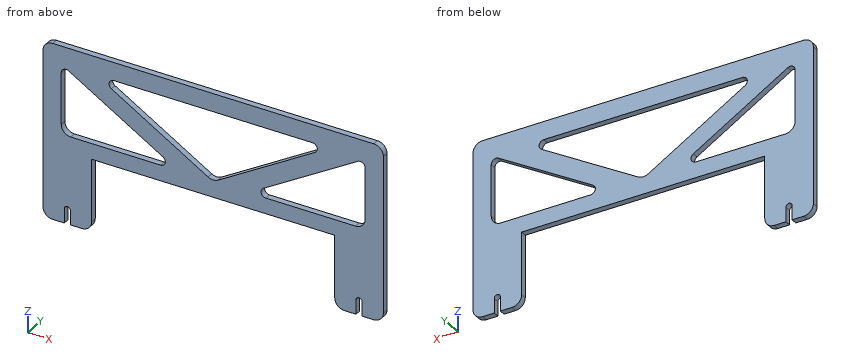
from build123d import *

# Parameters (mm, degrees)
SKETCH1_W           = 177.8
SKETCH1_H           = 67.31
BOSS_EXTRUDE1_DEPTH = 3.175
CUT_EXTRUDE1_DEPTH  = 4.175
CUT_EXTRUDE2_DEPTH  = 4.175
SKETCH5_W           = 127
SKETCH5_H           = 12.7
CUT_EXTRUDE3_DEPTH  = 4.175
FILLET1_R           = 5.08
FILLET2_R           = 2.54
SKETCH7_W           = 25.4
SKETCH7_H           = 38.1
BOSS_EXTRUDE2_DEPTH = 3.175
CUT_EXTRUDE4_DEPTH  = 4.175
FILLET3_R           = 5.08


with BuildPart() as part:
    # Sketch1 → Boss-Extrude1 (new body)
    with BuildSketch(Plane(origin=(0, 0, 0), x_dir=(1, 0, 0), z_dir=(0, 1, 0))):
        with Locations((88.9, 33.655)):
            Rectangle(SKETCH1_W, SKETCH1_H)
    extrude(amount=BOSS_EXTRUDE1_DEPTH)

    # Sketch3 → Cut-Extrude1 (cut, through all)
    with BuildSketch(Plane(origin=(0, 3.175, 0), x_dir=(1, 0, 0), z_dir=(0, 1, 0))):
        Polygon((88.9, 46.355), (27.943666175, 9.525), (149.856333825, 9.525), align=None)
        Polygon((9.525, 46.355), (9.525, 9.525), (70.481333825, 46.355), align=None)
        Polygon((168.275, 9.525), (107.318666175, 46.355), (168.275, 46.355), align=None)
    extrude(amount=-CUT_EXTRUDE1_DEPTH, mode=Mode.SUBTRACT)

    # Sketch4 → Cut-Extrude2 (cut, through all)
    with BuildSketch(Plane(origin=(0, 3.175, 0), x_dir=(1, 0, 0), z_dir=(0, 1, 0))):
        with BuildLine():
            Line((11.1125, 67.31), (11.1125, 62.23))
            ThreePointArc((11.1125, 62.23), (12.7, 60.6425), (14.2875, 62.23))
            Line((14.2875, 62.23), (14.2875, 67.31))
            Line((14.2875, 67.31), (11.1125, 67.31))
        make_face()
        with BuildLine():
            Line((166.6875, 67.31), (166.6875, 62.23))
            ThreePointArc((166.6875, 62.23), (165.1, 60.6425), (163.5125, 62.23))
            Line((163.5125, 62.23), (163.5125, 67.31))
            Line((163.5125, 67.31), (166.6875, 67.31))
        make_face()
    extrude(amount=-CUT_EXTRUDE2_DEPTH, mode=Mode.SUBTRACT)

    # Sketch5 → Cut-Extrude3 (cut, through all)
    with BuildSketch(Plane(origin=(0, 3.175, 0), x_dir=(1, 0, 0), z_dir=(0, 1, 0))):
        with Locations((88.9, 60.96)):
            Rectangle(SKETCH5_W, SKETCH5_H)
    extrude(amount=-CUT_EXTRUDE3_DEPTH, mode=Mode.SUBTRACT)

    # Fillet1
    fillet1_edges = [part.edges().sort_by_distance(p)[0] for p in [
        (88.9, 1.5875, -46.355),
        (9.525, 1.5875, -46.355),
        (168.275, 1.5875, -46.355),
        (0, 1.5875, -67.31),
        (177.8, 1.5875, -67.31),
        (177.8, 1.5875, 0),
        (0, 1.5875, 0),
        (25.4, 1.5875, -67.31),
        (152.4, 1.5875, -67.31),
    ]]
    fillet(fillet1_edges, radius=FILLET1_R)

    # Fillet2
    fillet2_edges = [part.edges().sort_by_distance(p)[0] for p in [
        (149.856333825, 1.5875, -9.525),
        (27.943666175, 1.5875, -9.525),
        (70.481333825, 1.5875, -46.355),
        (9.525, 1.5875, -9.525),
        (168.275, 1.5875, -9.525),
        (107.318666175, 1.5875, -46.355),
    ]]
    fillet(fillet2_edges, radius=FILLET2_R)

    # Sketch7 → Boss-Extrude2 (add)
    with BuildSketch(Plane(origin=(0, 3.175, 0), x_dir=(1, 0, 0), z_dir=(0, 1, 0))):
        with Locations((12.7, 73.66)):
            Rectangle(SKETCH7_W, SKETCH7_H)
        with Locations((165.1, 73.66)):
            Rectangle(SKETCH7_W, SKETCH7_H)
    extrude(amount=-BOSS_EXTRUDE2_DEPTH)

    # Sketch8 → Cut-Extrude4 (cut, through all)
    with BuildSketch(Plane(origin=(0, 3.175, 0), x_dir=(1, 0, 0), z_dir=(0, 1, 0))):
        with BuildLine():
            Line((11.1125, 92.71), (11.1125, 85.09))
            ThreePointArc((11.1125, 85.09), (12.7, 83.5025), (14.2875, 85.09))
            Line((14.2875, 85.09), (14.2875, 92.71))
            Line((14.2875, 92.71), (11.1125, 92.71))
        make_face()
        with BuildLine():
            Line((163.5125, 85.09), (163.5125, 92.71))
            Line((163.5125, 92.71), (166.6875, 92.71))
            Line((166.6875, 92.71), (166.6875, 85.09))
            ThreePointArc((166.6875, 85.09), (165.1, 83.5025), (163.5125, 85.09))
        make_face()
    extrude(amount=-CUT_EXTRUDE4_DEPTH, mode=Mode.SUBTRACT)

    # Fillet3
    fillet3_edges = [part.edges().sort_by_distance(p)[0] for p in [
        (25.4, 1.5875, -92.71),
        (0, 1.5875, -92.71),
        (177.8, 1.5875, -92.71),
        (152.4, 1.5875, -92.71),
    ]]
    fillet(fillet3_edges, radius=FILLET3_R)


solid = part.part
Build history of the part. All positions in model axes, mm. Round coordinates to 2 decimals unless told otherwise and drop trailing zeros. Loops run counter-clockwise (first coordinate to the right, second up) from the corner with the lowest first, then second, coordinate; pieces in that order, holes last. Notation, with made-up numbers: (-31.5, 70) -> (25.5, 70) arc R13 cw to (25.5, 85) -> close; hole circle Ø1 at (45.25, 60.25). An arc over 180 degrees is marked (long way). One line per item, written item: value. Start each with the question number.
Q1. Drop flat-ended pins along their axis: pin 1 Ø1.6 at (y, z) = (2, -90) entering from +X; pin 2 Ø1 at (x, y) = (146.5, 1) entering from -Z. Give the stop position or say it passes through.
Q2. Cut at B-B on x = 23. List the corners of the cut face in (y, z) (3 decimals).
Q3. Cut at A-A on z = -80.5. List the corners of the cut face in (x, y) (3 decimals).
Q4. Probe line 1 along Z through (x, y) = (89.5, 1.05) (3 decimals); line 2 along X through (y, z) = (0.95, -55); line 3 along X through (y, z) = (0.95, -84). List the from-to ranges inside material, lowest first.
Q5. Cut at D-D on x = 120.5. List the corners of the cut face in (y, z) (3 decimals), plus the area to 3 significant figures.
Q6. Cut at C-C on z = -16. List the corners of the cut face in (x, y) (3 decimals).
Computed:
1. pin 1: x = 177.55
1. pin 2: z = -54.61
2. outline: (0, -91.946) -> (3.175, -91.946) -> (3.175, -46.355) -> (0, -46.355) -> close; (0, -17.667) -> (3.175, -17.667) -> (3.175, 0) -> (0, 0) -> close
3. outline: (0, 0) -> (25.4, 0) -> (25.4, 3.175) -> (0, 3.175) -> close; (152.4, 0) -> (177.8, 0) -> (177.8, 3.175) -> (152.4, 3.175) -> close
4. line 1: -54.61 to -45.464, -9.525 to 0
4. line 2: 0 to 25.4, 152.4 to 177.8
4. line 3: 0 to 11.55, 13.85 to 25.4, 152.4 to 163.95, 166.25 to 177.8
5. outline: (0, -54.61) -> (3.175, -54.61) -> (3.175, -46.355) -> (0, -46.355) -> close; (0, -38.391) -> (3.175, -38.391) -> (3.175, -27.262) -> (0, -27.262) -> close; (0, -9.525) -> (3.175, -9.525) -> (3.175, 0) -> (0, 0) -> close
5. area: 91.8 mm²
6. outline: (0, 0) -> (9.525, 0) -> (9.525, 3.175) -> (0, 3.175) -> close; (20.242, 0) -> (38.66, 0) -> (38.66, 3.175) -> (20.242, 3.175) -> close; (139.14, 0) -> (157.558, 0) -> (157.558, 3.175) -> (139.14, 3.175) -> close; (168.275, 0) -> (177.8, 0) -> (177.8, 3.175) -> (168.275, 3.175) -> close
